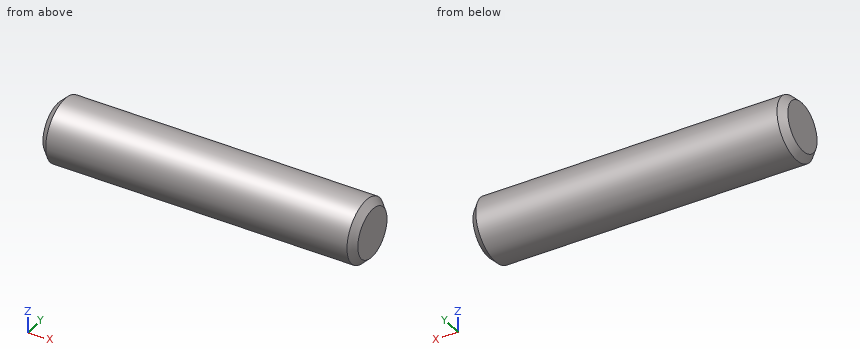
Autodesk Inventor part; units mm, degrees
ref_plane "Work Plane1" through (2.75, 0, 0) normal (0, -1, 0) x (1, 0, 0)
ref_plane "YZ Plane" through (0, 0, 0) normal (1, 0, 0) x (0, 1, 0)
ref_plane "XZ Plane" through (0, 0, 0) normal (0, 1, 0) x (-1, 0, 0)
sketch "Schizzo1" plane through (0, 0, 0) normal (0, 0, 1) x (1, 0, 0)
  line L0 (20, 4) -> (20, 0)
  line L1 (-20, 0) -> (20, 0)
  line L2 (-28, 0) -> (28, 0)
  line L3 (0, 4.8) -> (0, -0.8)
  line L4 (-20, 4) -> (-20, 0)
  line L5 (0, 4) -> (0, 0) construction
  line L6 (-28, 0) -> (28, 0)
  line L7 (-20, 4) -> (20, 4)
  dimension "d13" = 8
  dimension "d87" = 40
  dimension "d88" = 20
revolve "Corpo" add sketch "Schizzo1" angle 360 about axis through (-20, 0, 0) along (1, 0, 0)
thread "Filettatura1"
chamfer "Smusso1" distance 0.864 angle 45 1 edges at (20, -4, 0) measured on face at (-6.6667, 3.987, -0.3219)
chamfer "Smusso2" distance 0.864 angle 45 1 edges at (-20, -4, 0) measured on face at (-6.9547, 3.9482, -0.6416)
ref_plane "Work Plane1" through (2.75, 0, 0) normal (0, -1, 0) x (1, 0, 0)
equation "\"d13\" = NND"
equation "\"d87\" = NLG"
equation "\"d88\" = 0.5 * NLG"
equation "\"d1\" = GEL"
equation "\"d9\" = -0.5 * SPD + 0.5 * NND"
equation "\"d10\" = -0.5 * SPD + 0.5 * NND"
equation "\"d11\" = -0.5 * SPD + 0.5 * NND"
equation "\"d12\" = -0.5 * SPD + 0.5 * NND"
equation "\"NLG\" = 40"
equation "\"GEL\" = NLG"
equation "\"GAL\" = 0.61345 * PTC"
equation "\"SPD\" = 6.272"
equation "\"d0\" = NND"
equation "\"GUL\" = 0.61345 * PTC"
equation "\"NND\" = 8"
equation "\"GUL1\" = GUL"
equation "\"GAL1\" = GAL"
equation "\"d80\" = -GUL - GEL"
equation "\"d86\" = -GEL + GUL1"
equation "\"PTC\" = 1.25"
equation "\"THREADDIA\" = 8"
equation "\"TOA\" = 30deg"
equation "\"GD1\" = THREADDIA - 1.2269 * PTC"
properties part number "DIN 976-1 - M8 x 40 - B" material "Acciaio, Dolce"
Geometry: final body of the model. Coordinates: model frame, mm. Give positions to 0.01 mm unless a question says otherwise; leave off trailing zeros. Write each loop counter-clockwise with the first axis right and the second up, starting at its lowest first coordinate (ties: lowest second). Pieces come first, ordered by that corner, then holes. Notation, with made-up numbers: M -28,10.25 L -5,10.25 A23 ccw -5,46.25 Z; hole C -14,26.5 d9. An arc over 180 degrees is marked long. Answer in a Markdown table with one row per item. Add a question column.
(1) Ray query, line 1 (Z direction, x = 12.5, y = -0.25); line 2 (X direction, y = 0.25, z = 3.5). Return the intervals inside material, ascending.
(2) First-contact query: pin 1 (4 mm diameter, centred on x = -13.5, z = -2.5, fed in from +Y); pin 2 (2 mm diameter, centred on x = -4.5, y = 1.5, fed in from -Z). Flat tips, straight axial feed; report the tip coordinate or a pass-through.
(3) Section A-A on x = -12. Return loops of the section in (y, z), and give its area (3 significant figures).
Result set:
| question | item | result |
|---|---|---|
| 1 | line 1 | z = -3.99 to 3.99 |
| 1 | line 2 | x = -19.63 to 19.63 |
| 2 | pin 1 | stops at y = 3.97 |
| 2 | pin 2 | stops at z = -3.97 |
| 3 | outline | C 0,0 d8 |
| 3 | area | 50.3 mm^2 |
